Autodesk Inventor part; units mm, degrees
ref_plane "YZ Plane" through (0, 0, 0) normal (1, 0, 0) x (0, 1, 0)
ref_plane "XZ Plane" through (0, 0, 0) normal (0, 1, 0) x (-1, 0, 0)
ref_plane "XY Plane" through (0, 0, 0) normal (0, 0, 1) x (1, 0, 0)
sketch "Sketch1" plane through (0, 0, 0) normal (0, 0, 1) x (1, 0, 0)
  line L0 (0, 244.475) -> (19.05, 244.475)
  line L1 (19.05, 244.475) -> (19.05, 225.425)
  line L2 (19.05, 225.425) -> (0, 225.425)
  line L3 (0, 225.425) -> (0, 244.475)
  line L4 (19.05, 168.275) -> (0, 168.275)
  line L5 (0, 168.275) -> (0, 149.225)
  line L6 (0, 149.225) -> (19.05, 149.225)
  line L7 (19.05, 149.225) -> (19.05, 168.275)
  line L8 (0, 130.175) -> (19.05, 130.175)
  line L9 (19.05, 130.175) -> (19.05, 111.125)
  line L10 (19.05, 111.125) -> (0, 111.125)
  line L11 (0, 111.125) -> (0, 130.175)
  line L12 (0, 206.375) -> (19.05, 206.375)
  line L13 (19.05, 206.375) -> (19.05, 187.325)
  line L14 (19.05, 187.325) -> (0, 187.325)
  line L15 (0, 187.325) -> (0, 206.375)
  line L16 (0, 92.075) -> (19.05, 92.075)
  line L17 (19.05, 92.075) -> (19.05, 73.025)
  line L18 (19.05, 73.025) -> (0, 73.025)
  line L19 (0, 73.025) -> (0, 92.075)
  line L20 (0, 53.975) -> (19.05, 53.975)
  line L21 (19.05, 53.975) -> (19.05, 34.925)
  line L22 (19.05, 34.925) -> (0, 34.925)
  line L23 (0, 34.925) -> (0, 53.975)
  line L24 (0, 15.875) -> (19.05, 15.875)
  line L25 (19.05, 15.875) -> (19.05, -3.175)
  line L26 (19.05, -3.175) -> (0, -3.175)
  line L27 (0, -3.175) -> (0, 15.875)
  line L28 (0, 244.475) -> (206.375, 244.475)
  line L29 (206.375, 244.475) -> (206.375, 76.2)
  line L30 (206.375, 76.2) -> (0, 76.2)
  line L31 (19.05, 244.475) -> (19.05, 76.2)
  line L32 (206.375, 244.475) -> (19.05, 244.475)
  line L33 (19.05, 244.475) -> (19.05, 76.2)
  line L34 (19.05, 76.2) -> (206.375, 76.2)
  line L35 (206.375, 76.2) -> (206.375, 244.475)
  line L36 (0, 92.075) -> (19.05, 92.075)
  line L37 (19.05, 92.075) -> (19.05, 76.2)
  line L38 (19.05, 76.2) -> (0, 76.2)
  line L39 (0, 76.2) -> (0, 92.075)
  dimension "d0" = 19.05
  dimension "d1" = 19.05
  dimension "d3" = 19.05
  dimension "d4" = 19.05
  dimension "d5" = 19.05
  dimension "d6" = 19.05
  dimension "d7" = 19.05
  dimension "d8" = 19.05
  dimension "d9" = 19.05
  dimension "d10" = 19.05
  dimension "d11" = 19.05
  dimension "d12" = 19.05
  dimension "d13" = 19.05
  dimension "d14" = 19.05
  dimension "d15" = 19.05
  dimension "d16" = 19.05
  dimension "d17" = 19.05
  dimension "d18" = 19.05
  dimension "d19" = 19.05
  dimension "d21" = 206.375
  dimension "d22" = 168.275
  dimension "d23" = 206.375
extrude "Extrusion3" add sketch "Sketch1" along normal blind 19.05 contours L0 L1 L2 L3 | L28 L29 L30 L17 L31 L9 L7 L13 L1 | L13 L14 L15 L12 | L30 L19 L16 L17 | L7 L6 L5 L4 | L10 L11 L8 L9
mirror "Mirror2" about plane through (206.375, 76.2, 0) normal (1, 0, 0) of "Extrusion3"
sketch "Sketch3" plane through (0, 0, 19.05) normal (0, 0, 1) x (1, 0, 0)
  line L0 (0, 244.475) -> (412.75, 244.475)
  line L1 (19.05, 244.475) -> (393.7, 244.475)
  line L2 (393.7, 244.475) -> (393.7, 228.6)
  line L3 (393.7, 228.6) -> (19.05, 228.6)
  line L4 (19.05, 228.6) -> (19.05, 244.475)
  point P0 (0, 0)
  dimension "d33" = 15.875
extrude "Extrusion4" cut sketch "Sketch3" against normal blind 9.525
properties part number "deep_end" material "Wood (Birch)"
Geometry check sheet. Reference: the model listing, model coordinates, mm. A direction names the side the tool comes from. Give positions to 0.01 mm unless a question says otherwise; leave off trailing zeros. Order: outer loops, then holes, each group sorted by start corner. A loop starts at its lowest first (then second) coordinate and runs counter-clockwise, first axis right, second up.
1. Release check for a two-part mould opening along Y. For faces 5 (the face through (209, 76.2, 9)), 6 (the face through (9, 130.175, 9)), 7 (the face through (203, 162, 0)) record: pulls with the +Y half, pulls with the -Y half, needs draft (parallel to the pull), parting line crosses it, or undercut.
2. Thickness scan on L1, parallel to X at y = 238.5, z = 13; L2, parallel to X at y = 177.5, z = 15.5; L3, parallel to Y at x = 48, z = 11. Record the ranges inside material, lowest first.
3. Access from +Z, -Z, +X, -X, +Y, -Y to the whole of each face (thin tool, end or side, straight path). Record for faces 1 (the face through (393.7, 237, 14)), 2 (the face through (412.75, 197, 9)), 3 (the face through (19.05, 216, 9)), 4 (the face through (393.7, 101, 9)).
4. Section check A-A, the plane x = 133. Enter the section's corners in (y, z) (3 decimals).
5. Gauge pin test, flat ends, axial feed: pin 1 Ø3 at (y, z) = (95.5, 14) entering from +X; pin 2 Ø5.5 at (y, z) = (143, 13.5) entering from -X; pin 3 Ø1.5 at (x, z) = (224, 15) entering from +Y. Record the tip position at first contact, or that the pin passes through.
6. Section check B-B, the plane y = 144.5. Enter the section's corners in (x, z), and give its area (3 significant figures).
Values follow:
1. face 5: pulls with the -Y half
1. face 6: undercut
1. face 7: needs draft
2. L1: x = 0 to 19.05, 393.7 to 412.75
2. L2: x = 19.05 to 393.7
2. L3: y = 76.2 to 228.6
3. face 1: +Z, +Y
3. face 2: +Z, -Z, +X, +Y, -Y
3. face 3: +Z, -Z, -X
3. face 4: +Z, -Z, +X
4. outline: (76.2, 0) - (244.475, 0) - (244.475, 9.525) - (228.6, 9.525) - (228.6, 19.05) - (76.2, 19.05) - close
5. pin 1: stops at x = 393.7
5. pin 2: stops at x = 19.05
5. pin 3: stops at y = 228.6
6. outline: (19.05, 0) - (393.7, 0) - (393.7, 19.05) - (19.05, 19.05) - close
6. area: 7,140 mm2
